The listing builds one solid part. Answer for the finished solid, in the listing's coordinates (mm). Face numbers are marked on the shaded views. A direction names the side the tool comes from. Coordinates: 2 decimals unless noted, no trailing zeros. Write each loop counter-clockwise with the first axis right and the second up, starting at its lowest first coordinate (ties: lowest second). Pieces come first, ordered by that corner, then holes. Notation, with made-up numbers: M 51.25,56.25 L 80.25,56.25 A19 cw 80.25,61.25 Z; hole C 52,54 d1. An arc over 180 degrees is marked long. Put each result on its own line as item: value. Start each with the question number.
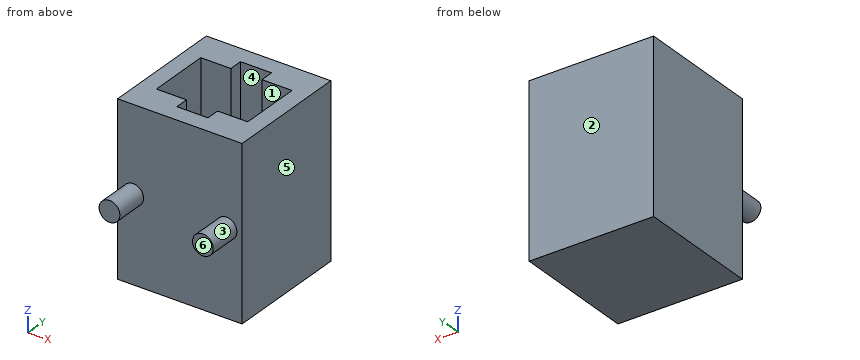
```python
from build123d import *

# Parameters (mm, degrees)
SKETCH1_W           = 15.24
SKETCH1_H           = 15.24
BOSS_EXTRUDE1_DEPTH = 20.828
CUT_EXTRUDE1_DEPTH  = 18.288
SKETCH3_R           = 1.27
BOSS_EXTRUDE2_DEPTH = 4.064


with BuildPart() as part:
    # Sketch1 → Boss-Extrude1 (new body)
    with BuildSketch(Plane.XY):
        Rectangle(SKETCH1_W, SKETCH1_H)
    extrude(amount=BOSS_EXTRUDE1_DEPTH)

    # Sketch2 → Cut-Extrude1 (cut)
    with BuildSketch(Plane.XY.offset(20.828)):
        Polygon((5.588, -3.81), (1.905, -3.81), (1.905, -5.461), (-1.905, -5.461), (-1.905, -3.81), (-5.588, -3.81), (-5.588, 3.81), (-1.905, 3.81), (-1.905, 5.461), (1.905, 5.461), (1.905, 3.81), (5.588, 3.81), align=None)
    extrude(amount=-CUT_EXTRUDE1_DEPTH, mode=Mode.SUBTRACT)

    # Sketch3 → Boss-Extrude2 (add)
    with BuildSketch(Plane.XZ.offset(7.62)):
        with Locations((-5.715, 10.414)):
            Circle(SKETCH3_R)
        with Locations((5.715, 10.414)):
            Circle(SKETCH3_R)
    extrude(amount=BOSS_EXTRUDE2_DEPTH)


solid = part.part
```
1) A cutting plane is placed at B-B on x = 0.5. Write down the section's boundary in (y, z).
2) A cutting plane is placed at D-D on z = 2.25. Write down the section's boundary in (x, y).
3) Given pin 1 Ø1.1 at (x, z) = (-3.5, 12) entering from -Y; pin 2 Ø2 at (y, z) = (-9.5, 4) entering from -X, each flat-ended and moving along its own axis, determine where each tip first touches the part or whether it passes through.
4) A cutting plane is placed at A-A on z = 14.5. Write down the section's boundary in (x, y) (3 decimals), then the cut area to 3 significant figures.
5) Determine the mould class of the marked faces 4, 5 and 6 for opening direction X: +X half, -X half, draft (parallel to the pull), parting line (faces both ways), or undercut.
6) For the marked faces 1, 2 and 3, determine the directions among +Z, -Z, +X, -X, +Y, -Y from which every point of the face is accessible in a straight line to the end or side of a thin tool.
7) Straight lines are drawn through the part: probe 1 along Y at (x, z) = (-2.75, 9); probe 2 along X at (y, z) = (-2.5, 5.5); probe 3 along Y at (x, z) = (-0.5, 5.75). For each, find the intervals that lie inside material, in ascending order.
8) A cutting plane is placed at C-C on y = 1. Write down the section's boundary in (x, z).
Answers follow:
1. outline: M -7.62,0 L 7.62,0 L 7.62,20.83 L 5.46,20.83 L 5.46,2.54 L -5.46,2.54 L -5.46,20.83 L -7.62,20.83 Z
2. outline: M -7.62,-7.62 L 7.62,-7.62 L 7.62,7.62 L -7.62,7.62 Z
3. pin 1: stops at y = -7.62
3. pin 2: passes through
4. outline: M -7.62,-7.62 L 7.62,-7.62 L 7.62,7.62 L -7.62,7.62 Z; hole M -5.588,-3.81 L -1.905,-3.81 L -1.905,-5.461 L 1.905,-5.461 L 1.905,-3.81 L 5.588,-3.81 L 5.588,3.81 L 1.905,3.81 L 1.905,5.461 L -1.905,5.461 L -1.905,3.81 L -5.588,3.81 Z
4. area: 135 mm²
5. face 4: undercut
5. face 5: +X half
5. face 6: draft
6. face 1: +Z
6. face 2: +Z, -Z, +X, -X, +Y
6. face 3: -Y
7. probe 1: y = -7.62 to -3.81, 3.81 to 7.62
7. probe 2: x = -7.62 to -5.59, 5.59 to 7.62
7. probe 3: y = -7.62 to -5.46, 5.46 to 7.62
8. outline: M -7.62,0 L 7.62,0 L 7.62,20.83 L 5.59,20.83 L 5.59,2.54 L -5.59,2.54 L -5.59,20.83 L -7.62,20.83 Z
